Read the model definition and answer for the solid it produces. Units are mm, in the model's axes. Face numbers are marked on the shaded views. A direction names the side the tool comes from. Give positions to 0.01 mm unless a question says otherwise; leave off trailing zeros. Write each loop counter-clockwise with the first axis right and the second up, starting at its lowest first coordinate (ties: lowest second). Pieces come first, ordered by that corner, then holes. Notation, with made-up numbers: (78.5, 2.5) -> (115.5, 2.5) arc R17 cw to (115.5, 20.5) -> close; hole circle Ø5 at (48.5, 60.25). An arc over 180 degrees is marked (long way). Use a Markdown table: item, result.
from build123d import *

# Parameters (mm, degrees)
F0_W     = 127
F0_H     = 127
F1_DEPTH = 50.8
F2_W     = 114.3
F2_H     = 38.1
F3_DEPTH = 127.001
F5_DEPTH = 50.801


with BuildPart() as f1:
    # F0 (on Top) → F1 (new body)
    with BuildSketch(Plane.XY):
        Rectangle(F0_W, F0_H)
    extrude(amount=F1_DEPTH)

    # F2 (on face) → F3 (cut, through all)
    with BuildSketch(Plane.XZ.offset(63.5)):
        with Locations((0, 25.4)):
            Rectangle(F2_W, F2_H)
    extrude(amount=-F3_DEPTH, mode=Mode.SUBTRACT)

    # F4 (on face) → F5 (cut, through all)
    with BuildSketch(Plane.XY.offset(50.8)):
        with BuildLine():
            ThreePointArc((50.8, -6.35), (44.45, 0), (50.8, 6.35))
            Line((50.8, 6.35), (-50.8, 6.35))
            ThreePointArc((-50.8, 6.35), (-46.309872, 4.490128), (-44.45, 0))
            ThreePointArc((-44.45, 0), (-46.309872, -4.490128), (-50.8, -6.35))
            Line((-50.8, -6.35), (50.8, -6.35))
        make_face()
        with BuildLine():
            ThreePointArc((50.8, -6.35), (55.290128, -4.490128), (57.15, 0))
            ThreePointArc((57.15, 0), (55.290128, 4.490128), (50.8, 6.35))
            ThreePointArc((50.8, 6.35), (44.45, 0), (50.8, -6.35))
        make_face()
        with BuildLine():
            ThreePointArc((-44.45, 0), (-46.309872, 4.490128), (-50.8, 6.35))
            ThreePointArc((-50.8, 6.35), (-55.290128, 4.490128), (-57.15, 0))
            ThreePointArc((-57.15, 0), (-55.290128, -4.490128), (-50.8, -6.35))
            ThreePointArc((-50.8, -6.35), (-46.309872, -4.490128), (-44.45, 0))
        make_face()
    extrude(amount=-F5_DEPTH, mode=Mode.SUBTRACT)


solid = f1.part
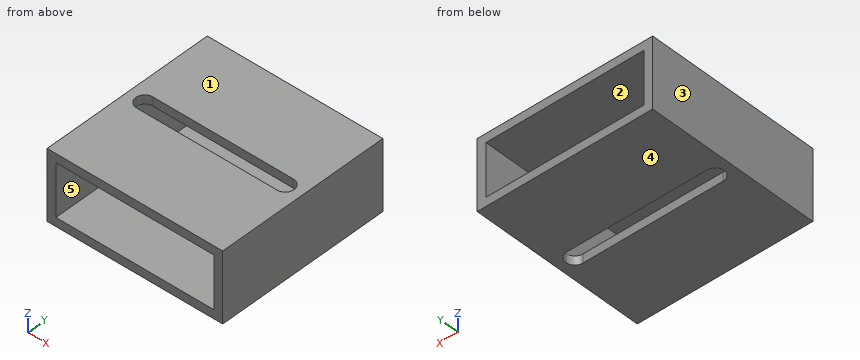
Item 1: A tool of negligible diameter and unlimited length cuts with its end or side. For the marked faces 4 and 5, from which of +Z, -Z, +X, -X, +Y, -Y can it reach the whole face along a straight path? Write none if from no direction.
Return value:
| item | result |
|---|---|
| face 4 | -Z, +X, -X, +Y, -Y |
| face 5 | +Y, -Y |
Item 2: For a pull along Z with two mould halves and no side action, classify the marked faces 1, 2 and 3 as +Z half, -Z half, draft (parallel to the pull), parting line (faces both ways), or undercut.
Return value:
| item | result |
|---|---|
| face 1 | +Z half |
| face 2 | undercut |
| face 3 | draft |
Item 3: A cutting plane is placed at C-C (y = -21.5). Give the vertices of the cut face in (x, z), then the cut area to 3 significant figures.
Return value:
| item | result |
|---|---|
| outline | (-63.5, 0) -> (63.5, 0) -> (63.5, 50.8) -> (-63.5, 50.8) -> close; hole (-57.15, 6.35) -> (57.15, 6.35) -> (57.15, 44.45) -> (-57.15, 44.45) -> close |
| area | 2,100 mm^2 |
Item 4: A cutting plane is placed at B-B (x = -16). Give the vertices of the cut face in (y, z), then the cut area to 3 significant figures.
Return value:
| item | result |
|---|---|
| outline | (-63.5, 0) -> (-6.35, 0) -> (-6.35, 6.35) -> (-63.5, 6.35) -> close; (-63.5, 44.45) -> (-6.35, 44.45) -> (-6.35, 50.8) -> (-63.5, 50.8) -> close; (6.35, 0) -> (63.5, 0) -> (63.5, 6.35) -> (6.35, 6.35) -> close; (6.35, 44.45) -> (63.5, 44.45) -> (63.5, 50.8) -> (6.35, 50.8) -> close |
| area | 1,450 mm^2 |
Item 5: Straight lines are drawn through the part: line 1 along X through (y, z) = (-0.5, 47.5); line 2 along X through (y, z) = (-3, 25); line 3 along Z through (x, y) = (-44, -46). For each, find the intervals that lie inside material, in ascending order. Write a range as [from, to].
Return value:
| item | result |
|---|---|
| line 1 | [-63.5, -57.13], [57.13, 63.5] |
| line 2 | [-63.5, -57.15], [57.15, 63.5] |
| line 3 | [0, 6.35], [44.45, 50.8] |
Item 6: A cutting plane is placed at D-D (y = -3.5). Give the vertices of the cut face in (x, z), then the cut area to 3 significant figures.
Return value:
| item | result |
|---|---|
| outline | (-63.5, 0) -> (-56.1, 0) -> (-56.1, 6.35) -> (-57.15, 6.35) -> (-57.15, 44.45) -> (-56.1, 44.45) -> (-56.1, 50.8) -> (-63.5, 50.8) -> close; (56.1, 0) -> (63.5, 0) -> (63.5, 50.8) -> (56.1, 50.8) -> (56.1, 44.45) -> (57.15, 44.45) -> (57.15, 6.35) -> (56.1, 6.35) -> close |
| area | 672 mm^2 |
Item 7: A cutting plane is placed at A-A (z = 23). Give the vertices of the cut face in (x, y).
Return value:
| item | result |
|---|---|
| outline | (-63.5, -63.5) -> (-57.15, -63.5) -> (-57.15, 63.5) -> (-63.5, 63.5) -> close; (57.15, -63.5) -> (63.5, -63.5) -> (63.5, 63.5) -> (57.15, 63.5) -> close |
